Design review of the part shown in the three views and the two pictorial views. Dimensions are in mm from the part's minimum x, y and z. A direction names the side the tool comes from. Give positions to 0.01 mm unless a question says otherwise; leave off trailing zeros. Loops run counter-clockwise (first coordinate to the right, second up) from the corner with the lowest first, then second, coordinate; pieces in that order, holes last.
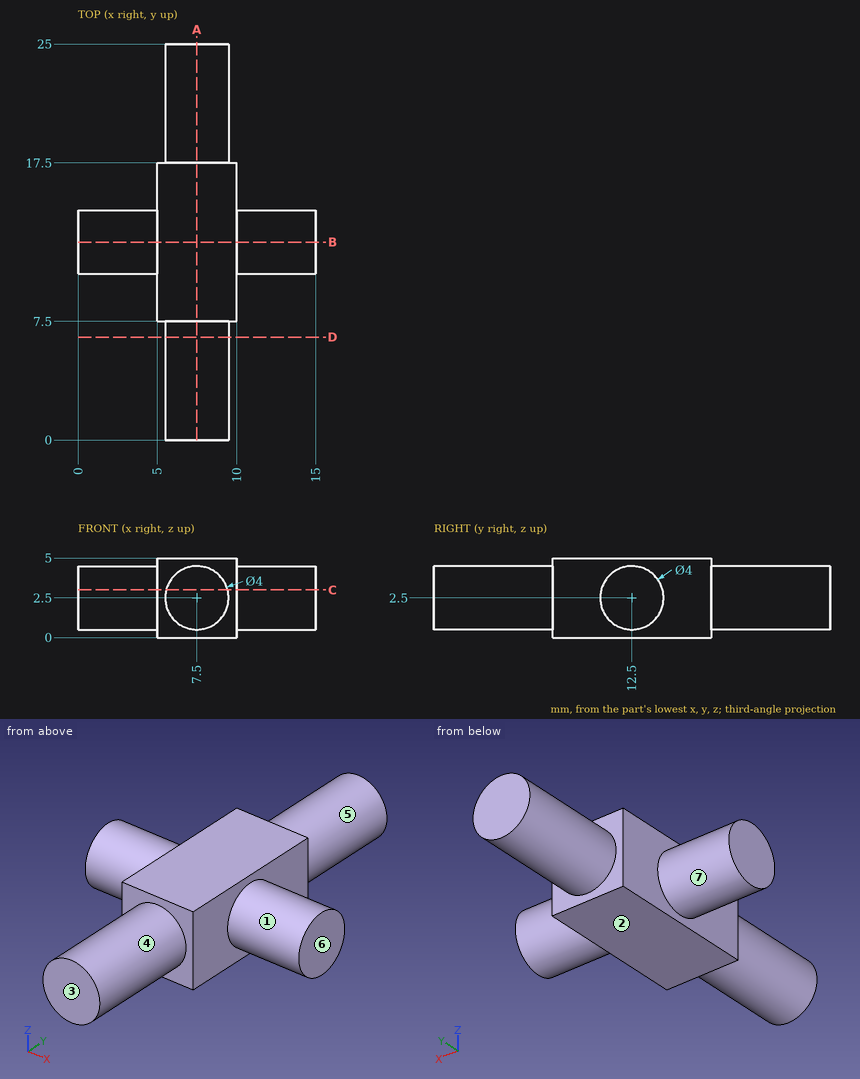
Q1. Take a section at D-D (y = 6.5). Give the boundary of the cut face in (x, z), plus the area to 3 significant figures.
Results:
outline: circle Ø4 at (7.5, 2.5)
area: 12.6 mm2
Q2. Draft analysis for pull direction Y (two halves, no side actions). For the marked faces 1, 2 and 3, state which applies: pulls with the +Y half, pulls with the -Y half, needs draft (parallel to the pull), parting line crosses it, or undercut.
Results:
face 1: parting line crosses it
face 2: needs draft
face 3: pulls with the -Y half
Q3. Tool access review of the marked faces 4, 5, 6 and 7: name each direction out of +Z, -Z, +X, -X, +Y, -Y from which nothing blocks a thin tool from reaching the whole face with its end or side.
Results:
face 4: -Y
face 5: +Y
face 6: +Z, -Z, +X, +Y, -Y
face 7: -X
Q4. Take a section at B-B (y = 12.5). Give the boundary of the cut face in (x, z), plus the area to 3 significant figures.
Results:
outline: (0, 0.5) - (5, 0.5) - (5, 0) - (10, 0) - (10, 0.5) - (15, 0.5) - (15, 4.5) - (10, 4.5) - (10, 5) - (5, 5) - (5, 4.5) - (0, 4.5) - close
area: 65.0 mm2
Q5. Wall thickness on line 1 (X direction, y = 10.5, z = 1.45); line 2 (Z direction, x = 7.5, y = 19.5); line 3 (Y direction, x = 9.5, z = 1.4): over which ranges is each line inside the solid? List them lowest first.
Results:
line 1: x = 5 to 10
line 2: z = 0.5 to 4.5
line 3: y = 7.5 to 17.5
Q6. Take a section at C-C (z = 3). Give the boundary of the cut face in (x, y), plus the area to 3 significant figures.
Results:
outline: (0, 10.56) - (5, 10.56) - (5, 7.5) - (5.56, 7.5) - (5.56, 0) - (9.44, 0) - (9.44, 7.5) - (10, 7.5) - (10, 10.56) - (15, 10.56) - (15, 14.44) - (10, 14.44) - (10, 17.5) - (9.44, 17.5) - (9.44, 25) - (5.56, 25) - (5.56, 17.5) - (5, 17.5) - (5, 14.44) - (0, 14.44) - close
area: 147 mm2
Q7. Take a section at A-A (x = 7.5). Give the boundary of the cut face in (y, z), plus the area to 3 significant figures.
Results:
outline: (0, 0.5) - (7.5, 0.5) - (7.5, 0) - (17.5, 0) - (17.5, 0.5) - (25, 0.5) - (25, 4.5) - (17.5, 4.5) - (17.5, 5) - (7.5, 5) - (7.5, 4.5) - (0, 4.5) - close
area: 110 mm2
Q8. Insertion check: pin 1 (2 mm diameter, centred on x = 5, y = 19, fed in from +Z); pin 2 (4 mm diameter, centred on x = 2.5, y = 9.5, fed in from -Z); pin 3 (1 mm diameter, centred on y = 11, z = 4, fed in from -X); pin 4 (1 mm diameter, centred on y = 16.5, z = 1.5, fed in from +X). Each pin has a flat end and moves straight along its axis. Give the tip position at first contact, or say it passes through.
Results:
pin 1: stops at z = 3.82
pin 2: stops at z = 0.77
pin 3: stops at x = 0
pin 4: stops at x = 10
